Verification items for the finished model (mm, model axes). A direction names the side the tool comes from. Give positions to 0.01 mm unless a question says otherwise; leave off trailing zeros. Write each loop counter-clockwise with the first axis right and the second up, starting at its lowest first coordinate (ties: lowest second). Pieces come first, ordered by that corner, then holes. Notation, with made-up numbers: (36, -17) -> (86, -17) arc R17 cw to (86, -1) -> close; hole circle Ø5 at (27.5, 77.5). An arc over 180 degrees is marked (long way). Use CSV: the item, a comma, the result in double quotes. Start each with the question number.
```python
from build123d import *

# Parameters (mm, degrees)
F1_DEPTH  = 100
F2_R      = 21.59
F4_DEPTH  = 52
F3_R      = 21.59
F5_DEPTH  = 52
F6_DEPTH  = 2.5
F7_DEPTH  = 95
F8_DEPTH  = 2.5
F3_R_2    = 24
F9_DEPTH  = 51
F10_START = 43.5
F10_DEPTH = 5
F11_START = 43.5
F11_DEPTH = 5
F2_R_2    = 24
F12_DEPTH = 52


# Not quite as in the source:
# - a feature names something its author has since deleted; it is built from what else it names


with BuildPart() as f1:
    # F0 (on Front) → F1 (new body, symmetric)
    with BuildSketch(Plane.XZ):
        Polygon((-80, 0), (-55.6696653366, -55), (-51.7864015908, -55), (-51.7864015908, -38.9201976359), (-18.3995570987, -3.0922384467), (18.3995570987, -3.0922384467), (51.7864015908, -38.9201976359), (51.7864015908, -55), (55.6696653366, -55), (80, 0), (45, 35), (-45, 35), align=None)
        with BuildLine():
            Line((-18.3995570987, -3.0922384467), (-51.7864015908, -38.9201976359))
            Line((-51.7864015908, -38.9201976359), (-12.7, -38.9201976359))
            ThreePointArc((-12.7, -38.9201976359), (0, -26.2201976359), (12.7, -38.9201976359))
            Line((12.7, -38.9201976359), (51.7864015908, -38.9201976359))
            Line((51.7864015908, -38.9201976359), (18.3995570987, -3.0922384467))
            Line((18.3995570987, -3.0922384467), (-18.3995570987, -3.0922384467))
        make_face()
        with BuildLine():
            Line((-51.7864015908, -38.9201976359), (-51.7864015908, -55))
            Line((-51.7864015908, -55), (51.7864015908, -55))
            Line((51.7864015908, -55), (51.7864015908, -38.9201976359))
            Line((51.7864015908, -38.9201976359), (12.7, -38.9201976359))
            ThreePointArc((12.7, -38.9201976359), (0, -51.6201976359), (-12.7, -38.9201976359))
            Line((-12.7, -38.9201976359), (-51.7864015908, -38.9201976359))
        make_face()
    extrude(amount=F1_DEPTH, both=True)

    # F2 (on face) → F4 (cut)
    with BuildSketch(Plane(origin=(40, 0, 40), x_dir=(0, 1, 0), z_dir=(0.7071067812, 0, 0.7071067812))):
        with Locations((72.954, -31.8198008825)):
            Circle(F2_R)
        with Locations((24.318, -31.8198008825)):
            Circle(F2_R)
        with Locations((-24.318, -31.8198008824)):
            Circle(F2_R)
        with Locations((-72.954, -31.8198008825)):
            Circle(F2_R)
    extrude(amount=-F4_DEPTH, mode=Mode.SUBTRACT)

    # F3 (on face) → F5 (cut)
    with BuildSketch(Plane(origin=(-40, 0, 40), x_dir=(0, -1, 0), z_dir=(-0.7071067812, 0, 0.7071067812))):
        with Locations((-72.9539923101, -31.8285424949)):
            Circle(F3_R)
        with Locations((-24.3179954494, -31.8110678119)):
            Circle(F3_R)
        with Locations((24.3180014113, -31.8285424949)):
            Circle(F3_R)
        with Locations((72.9540014113, -31.8285424949)):
            Circle(F3_R)
    extrude(amount=-F5_DEPTH, mode=Mode.SUBTRACT)

    # F0 (on Front) → F6 (join, symmetric)
    with BuildSketch(Plane.XZ):
        with BuildLine():
            Line((-18.3995570987, -3.0922384467), (-51.7864015908, -38.9201976359))
            Line((-51.7864015908, -38.9201976359), (-12.7, -38.9201976359))
            ThreePointArc((-12.7, -38.9201976359), (0, -26.2201976359), (12.7, -38.9201976359))
            Line((12.7, -38.9201976359), (51.7864015908, -38.9201976359))
            Line((51.7864015908, -38.9201976359), (18.3995570987, -3.0922384467))
            Line((18.3995570987, -3.0922384467), (-18.3995570987, -3.0922384467))
        make_face()
    extrude(amount=F6_DEPTH, both=True)

    # F0 (on Front) → F7 (cut, symmetric)
    with BuildSketch(Plane.XZ):
        with BuildLine():
            Line((-18.3995570987, -3.0922384467), (-51.7864015908, -38.9201976359))
            Line((-51.7864015908, -38.9201976359), (-12.7, -38.9201976359))
            ThreePointArc((-12.7, -38.9201976359), (0, -26.2201976359), (12.7, -38.9201976359))
            Line((12.7, -38.9201976359), (51.7864015908, -38.9201976359))
            Line((51.7864015908, -38.9201976359), (18.3995570987, -3.0922384467))
            Line((18.3995570987, -3.0922384467), (-18.3995570987, -3.0922384467))
        make_face()
        with BuildLine():
            Line((-51.7864015908, -38.9201976359), (-51.7864015908, -55))
            Line((-51.7864015908, -55), (51.7864015908, -55))
            Line((51.7864015908, -55), (51.7864015908, -38.9201976359))
            Line((51.7864015908, -38.9201976359), (12.7, -38.9201976359))
            ThreePointArc((12.7, -38.9201976359), (0, -51.6201976359), (-12.7, -38.9201976359))
            Line((-12.7, -38.9201976359), (-51.7864015908, -38.9201976359))
        make_face()
    extrude(amount=F7_DEPTH, both=True, mode=Mode.SUBTRACT)

    # F0 (on Front) → F8 (join, symmetric)
    with BuildSketch(Plane.XZ):
        with BuildLine():
            Line((-18.3995570987, -3.0922384467), (-51.7864015908, -38.9201976359))
            Line((-51.7864015908, -38.9201976359), (-12.7, -38.9201976359))
            ThreePointArc((-12.7, -38.9201976359), (0, -26.2201976359), (12.7, -38.9201976359))
            Line((12.7, -38.9201976359), (51.7864015908, -38.9201976359))
            Line((51.7864015908, -38.9201976359), (18.3995570987, -3.0922384467))
            Line((18.3995570987, -3.0922384467), (-18.3995570987, -3.0922384467))
        make_face()
    extrude(amount=F8_DEPTH, both=True)



with BuildPart() as f9:
    # F3 (on face) → F9 (new body)
    with BuildSketch(Plane(origin=(-40, 0, 40), x_dir=(0, -1, 0), z_dir=(-0.7071067812, 0, 0.7071067812))):
        with Locations((24.3180014113, -31.8285424949)):
            Circle(F3_R_2)
        with Locations((24.3180014113, -31.8285424949)):
            Circle(F3_R, mode=Mode.SUBTRACT)
    extrude(amount=-F9_DEPTH)


with BuildPart() as f9b:
    # F3 (on face) → F9, piece 2 (new body)
    with BuildSketch(Plane(origin=(-40, 0, 40), x_dir=(0, -1, 0), z_dir=(-0.7071067812, 0, 0.7071067812))):
        with Locations((72.9540014113, -31.8285424949)):
            Circle(F3_R_2)
        with Locations((72.9540014113, -31.8285424949)):
            Circle(F3_R, mode=Mode.SUBTRACT)
    extrude(amount=-F9_DEPTH)


with BuildPart() as f9c:
    # F3 (on face) → F9, piece 3 (new body)
    with BuildSketch(Plane(origin=(-40, 0, 40), x_dir=(0, -1, 0), z_dir=(-0.7071067812, 0, 0.7071067812))):
        with Locations((-24.3180014113, -31.8285424949)):
            Circle(F3_R_2)
        with Locations((-24.3179954494, -31.8110678119)):
            Circle(F3_R, mode=Mode.SUBTRACT)
    extrude(amount=-F9_DEPTH)


with BuildPart() as f9d:
    # F3 (on face) → F9, piece 4 (new body)
    with BuildSketch(Plane(origin=(-40, 0, 40), x_dir=(0, -1, 0), z_dir=(-0.7071067812, 0, 0.7071067812))):
        with Locations((-72.9540014113, -31.8285424949)):
            Circle(F3_R_2)
        with Locations((-72.9539923101, -31.8285424949)):
            Circle(F3_R, mode=Mode.SUBTRACT)
    extrude(amount=-F9_DEPTH)


with BuildPart() as f1_1:
    add(f1.part)

    add(f9.part)  # F10 merges F9

    add(f9b.part)  # F10 merges F9b
    # F8_face (on face) → F10 (join)
    with BuildSketch(Plane(origin=(0, -2.5, -22.7617883235), x_dir=(1, 0, 0), z_dir=(0, -1, 0)).offset(F10_START)):
        with BuildLine():
            Line((-18.3995570987, 19.6695498768), (-51.7864015908, -16.1584093124))
            Line((-51.7864015908, -16.1584093124), (-12.7, -16.1584093124))
            ThreePointArc((-12.7, -16.1584093124), (0, -3.4584093124), (12.7, -16.1584093124))
            Line((12.7, -16.1584093124), (51.7864015908, -16.1584093124))
            Line((51.7864015908, -16.1584093124), (18.3995570987, 19.6695498768))
            Line((18.3995570987, 19.6695498768), (-18.3995570987, 19.6695498768))
        make_face()
    extrude(amount=F10_DEPTH)


    add(f9c.part)  # F11 merges F9c

    add(f9d.part)  # F11 merges F9d
    # F8_face1 (on face) → F11 (join)
    with BuildSketch(Plane(origin=(0, 2.5, -22.7617883235), x_dir=(1, 0, 0), z_dir=(0, 1, 0)).offset(F11_START)):
        with BuildLine():
            Line((-51.7864015908, 16.1584093124), (-18.3995570987, -19.6695498768))
            Line((-18.3995570987, -19.6695498768), (18.3995570987, -19.6695498768))
            Line((18.3995570987, -19.6695498768), (51.7864015908, 16.1584093124))
            Line((51.7864015908, 16.1584093124), (12.7, 16.1584093124))
            ThreePointArc((12.7, 16.1584093124), (0, 3.4584093124), (-12.7, 16.1584093124))
            Line((-12.7, 16.1584093124), (-51.7864015908, 16.1584093124))
        make_face()
    extrude(amount=F11_DEPTH)


with BuildPart() as f12:
    # F2 (on face) → F12 (new body)
    with BuildSketch(Plane(origin=(40, 0, 40), x_dir=(0, 1, 0), z_dir=(0.7071067812, 0, 0.7071067812))):
        with Locations((-72.954, -31.8198008825)):
            Circle(F2_R_2)
        with Locations((-72.954, -31.8198008825)):
            Circle(F2_R, mode=Mode.SUBTRACT)
    extrude(amount=-F12_DEPTH)


with BuildPart() as f12b:
    # F2 (on face) → F12, piece 2 (new body)
    with BuildSketch(Plane(origin=(40, 0, 40), x_dir=(0, 1, 0), z_dir=(0.7071067812, 0, 0.7071067812))):
        with Locations((-24.318, -31.8198008824)):
            Circle(F2_R_2)
        with Locations((-24.318, -31.8198008824)):
            Circle(F2_R, mode=Mode.SUBTRACT)
    extrude(amount=-F12_DEPTH)


with BuildPart() as f12c:
    # F2 (on face) → F12, piece 3 (new body)
    with BuildSketch(Plane(origin=(40, 0, 40), x_dir=(0, 1, 0), z_dir=(0.7071067812, 0, 0.7071067812))):
        with Locations((24.318, -31.8198008825)):
            Circle(F2_R_2)
        with Locations((24.318, -31.8198008825)):
            Circle(F2_R, mode=Mode.SUBTRACT)
    extrude(amount=-F12_DEPTH)


with BuildPart() as f12d:
    # F2 (on face) → F12, piece 4 (new body)
    with BuildSketch(Plane(origin=(40, 0, 40), x_dir=(0, 1, 0), z_dir=(0.7071067812, 0, 0.7071067812))):
        with Locations((72.954, -31.8198008825)):
            Circle(F2_R_2)
        with Locations((72.954, -31.8198008825)):
            Circle(F2_R, mode=Mode.SUBTRACT)
    extrude(amount=-F12_DEPTH)


with BuildPart() as f1_2:
    add(f1_1.part)

    # F13: union F12b, F12, F12d, F12c
    add(f12b.part)
    add(f12.part)
    add(f12d.part)
    add(f12c.part)


solid = f1_2.part
```
(1) Draft check along Z on faces 4 (the face through (-41.536, -19.315, -33.661)), 5 (the face through (-19.57, 44.75, -4.35)), 6 (the face through (-17.12, -91.47, -6.3)). Enter one of: released by +Z, released by -Z, zero draft, split by the parting line, or undercut.
(2) Thickness scan on line 1 (Z direction, x = 0, y = -98); line 2 (X direction, y = -8, z = -8); line 3 (X direction, y = -88, z = 5.5). Record the ranges inside material, lowest first. Write a range as from..to.
(3) Go/stop test with flat-tipped pins: pin 1 (10 mm diameter, centred on y = 44, z = -41, fed in from +X); pin 2 (20.5 mm diameter, centred on x = 0, z = -38.92, fed in from +Y); pin 3 (5.5 mm diameter, centred on x = -24.5, y = -49.5, fed in from -Z); pin 4 (18.5 mm diameter, centred on x = 9, y = 69, fed in from -Z). Record where each tip stops, or that it passes through.
(4) Section check C-C on z = -16. Give the number of separate pieces and of enclosed holes in the cut face, then the cut area to 3 significant figures.
(5) Set-up check for faces 1 (the face through (-16.98, 91.31, -6.17)), 2 (the face through (-1.653, -97.535, -51.512)), 3 (the face through (47.569, -73.308, -34.394)): record each of +Z, -Z, +X, -X, +Y, -Y from which the full face is reachable in a straight line by a thin tool's end or side.
(6) Section check A-A on x = 0. Record the cut outline in (y, z), then the cut area to 3 significant figures.
(7) Section check B-B on y = 36.5. Record the cut outline in (x, z), then the cut area to 3 significant figures.
Data:
1,face 4,"released by -Z"
1,face 5,"undercut"
1,face 6,"undercut"
2,line 1,"z = -55..-51.62, -26.22..35"
2,line 2,"x = -76.46..-57, -17.02..-15.88, 14.46..17.01, 56.99..76.46"
2,line 3,"x = -74.5..-72.41, -28.62..28.6, 72.4..74.5"
3,pin 1,"stops at x = 64.07"
3,pin 2,"passes through"
3,pin 3,"stops at z = -38.92"
3,pin 4,"stops at z = -6.69"
4,separate pieces,"1"
4,enclosed holes,"4"
4,area,"10,800 mm2"
5,face 1,"none"
5,face 2,"+Y, -Y"
5,face 3,"-Z"
6,outline,"(-100, -55) -> (-95, -55) -> (-95, -51.62) -> (-100, -51.62) -> close; (-100, -26.22) -> (-95, -26.22) -> (-95, -3.09) -> (-51, -3.09) -> (-51, -26.22) -> (-46, -26.22) -> (-46, -3.09) -> (-2.5, -3.09) -> (-2.5, -26.22) -> (2.5, -26.22) -> (2.5, -3.09) -> (46, -3.09) -> (46, -26.22) -> (51, -26.22) -> (51, -3.09) -> (95, -3.09) -> (95, -26.22) -> (100, -26.22) -> (100, 35) -> (-100, 35) -> close; (95, -55) -> (100, -55) -> (100, -51.62) -> (95, -51.62) -> close"
6,area,"8,230 mm2"
7,outline,"(-80, 0) -> (-55.67, -55) -> (-51.79, -55) -> (-51.79, -38.92) -> (-43.85, -30.4) -> (-41.07, -33.19) -> (-39.04, -31.16) -> (-75.1, 4.9) -> close; (-49.89, 30.11) -> (-13.83, -5.95) -> (-11.82, -3.95) -> (-12.68, -3.09) -> (12.66, -3.09) -> (11.11, -4.65) -> (13.13, -6.67) -> (49.9, 30.1) -> (45, 35) -> (-45, 35) -> close; (38.33, -31.87) -> (40.35, -33.89) -> (43.85, -30.4) -> (51.79, -38.92) -> (51.79, -55) -> (55.67, -55) -> (80, 0) -> (75.1, 4.9) -> close"
7,area,"4,400 mm2"
